Read the model definition and answer for the solid it produces. Units are mm, in the model's axes. Give positions to 0.01 mm unless a question says otherwise; leave off trailing zeros. Order: outer loops, then holes, each group sorted by start corner. A loop starts at its lowest first (then second) coordinate and runs counter-clockwise, first axis right, second up.
Item 1: Given pin 1 Ø2 at (x, z) = (31.61, 18.25) entering from +Y; pin 2 Ø18 at (x, z) = (-250, 0) entering from +Y, each flat-ended and moving along its own axis, determine where each tip first touches the part or whether it passes through.
Item 2: A cutting plane is placed at B-B (y = 6.35). State how many separate pieces and enclosed holes the cut face has, plus the area to 3 significant figures.
Item 3: A cutting plane is placed at C-C (x = -226). Write down the section's boundary in (y, z).
Item 4: Find the intervals of material crossed by line 1 along Z through (x, y) = (-169.5, 6.4); line 2 along Z through (x, y) = (-73.5, 6.9); line 3 along Z through (x, y) = (-159.5, 7.2), in increasing order.
Item 5: A cutting plane is placed at A-A (x = 5.5). Write down the section's boundary in (y, z).
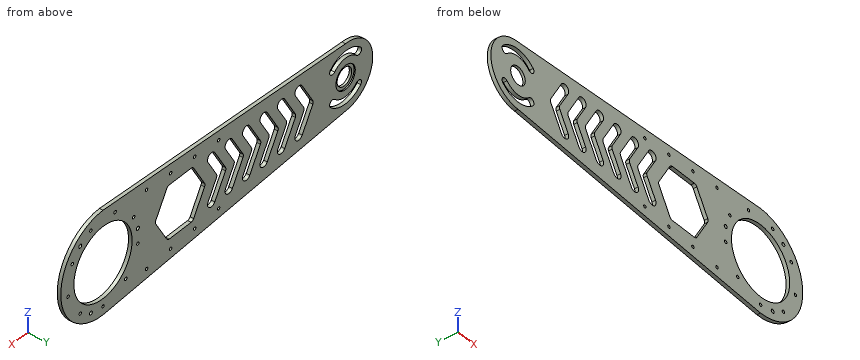
from build123d import *

# Parameters (mm, degrees)
EXTRUDE_1_DEPTH     = 3
SKETCH_3_R          = 1.25
SKETCH_3_R_2        = 30
SKETCH_3_R_3        = 1.5
CUT_EXTRUDE_1_DEPTH = 3
CUT_EXTRUDE_2_DEPTH = 3
SKETCH_5_R          = 1.25
CUT_EXTRUDE_3_DEPTH = 10
SKETCH_6_R          = 10
CUT_EXTRUDE_4_DEPTH = 1
SKETCH_7_R          = 7.5
CUT_EXTRUDE_5_DEPTH = 11


with BuildPart() as part:
    # 草图2 → 凸台-拉伸1 (new body)
    with BuildSketch(Plane(origin=(0, 5, 0), x_dir=(1, 0, 0), z_dir=(0, 1, 0))):
        with BuildLine():
            Line((-250, 28), (0, 43.5))
            ThreePointArc((0, 43.5), (43.5, 0), (0, -43.5))
            Line((0, -43.5), (-250, -28))
            ThreePointArc((-250, -28), (-278, 0), (-250, 28))
        make_face()
    extrude(amount=EXTRUDE_1_DEPTH)

    # 草图3 → 切除-拉伸1 (cut)
    with BuildSketch(Plane(origin=(0, 8, 0), x_dir=(1, 0, 0), z_dir=(0, 1, 0))):
        with Locations(Location((-250, 4, 0), (0, 0, 270))):
            Circle(SKETCH_3_R)
        with Locations(Location((-246, 0, 0), (0, 0, 270))):
            Circle(SKETCH_3_R)
        with Locations(Location((-250, -4, 0), (0, 0, 270))):
            Circle(SKETCH_3_R)
        with Locations(Location((-254, 0, 0), (0, 0, 270))):
            Circle(SKETCH_3_R)
        with Locations(Location((0, 0, 0), (0, 0, 270))):
            Circle(SKETCH_3_R_2)
        with Locations(Location((0, 36.5, 0), (0, 0, 270))):
            Circle(SKETCH_3_R)
        with Locations(Location((12.483735231, 34.298780659, 0), (0, 0, 270))):
            Circle(SKETCH_3_R_3)
        with Locations(Location((23.461747754, 27.960622174, 0), (0, 0, 270))):
            Circle(SKETCH_3_R)
        with Locations(Location((-23.461747754, 27.960622174, 0), (0, 0, 270))):
            Circle(SKETCH_3_R)
        with Locations(Location((-35.945482985, 6.338158485, 0), (0, 0, 270))):
            Circle(SKETCH_3_R)
        with Locations(Location((-35.945482985, -6.338158485, 0), (0, 0, 270))):
            Circle(SKETCH_3_R_3)
        with Locations(Location((-31.609927238, -18.25, 0), (0, 0, 270))):
            Circle(SKETCH_3_R)
        with Locations(Location((-12.483735231, -34.298780659, 0), (0, 0, 270))):
            Circle(SKETCH_3_R)
        with Locations(Location((12.483735231, -34.298780659, 0), (0, 0, 270))):
            Circle(SKETCH_3_R)
        with Locations(Location((23.461747754, -27.960622174, 0), (0, 0, 270))):
            Circle(SKETCH_3_R_3)
        with Locations(Location((31.609927238, -18.25, 0), (0, 0, 270))):
            Circle(SKETCH_3_R)
        with Locations(Location((35.945482985, 6.338158485, 0), (0, 0, 270))):
            Circle(SKETCH_3_R)
        with BuildLine():
            ThreePointArc((-265.553651429, 15.553651429), (-265.553651429, 11.316406256), (-261.316406256, 11.316406256))
            ThreePointArc((-261.316406256, 11.316406256), (-250, 16.003815204), (-238.683593744, 11.316406256))
            ThreePointArc((-238.683593744, 11.316406256), (-234.446348571, 11.316406256), (-234.446348571, 15.553651429))
            ThreePointArc((-234.446348571, 15.553651429), (-250, 21.996184796), (-265.553651429, 15.553651429))
        make_face()
        with BuildLine():
            ThreePointArc((-261.316406256, -11.316406256), (-250, -16.003815204), (-238.683593744, -11.316406256))
            ThreePointArc((-238.683593744, -11.316406256), (-234.446348571, -11.316406256), (-234.446348571, -15.553651429))
            ThreePointArc((-234.446348571, -15.553651429), (-250, -21.996184796), (-265.553651429, -15.553651429))
            ThreePointArc((-265.553651429, -15.553651429), (-265.553651429, -11.316406256), (-261.316406256, -11.316406256))
        make_face()
    extrude(amount=-CUT_EXTRUDE_1_DEPTH, mode=Mode.SUBTRACT)

    # 草图4 → 切除-拉伸2 (cut)
    with BuildSketch(Plane(origin=(0, 8, 0), x_dir=(1, 0, 0), z_dir=(0, 1, 0))):
        with BuildLine():
            Line((-216.23889617, 1.5), (-205.267472927, 20.503062488))
            ThreePointArc((-205.267472927, 20.503062488), (-199.762485666, 21.978119379), (-198.287428775, 16.473132117))
            Line((-198.287428775, 16.473132117), (-206.932170633, 1.5))
            ThreePointArc((-206.932170633, 1.5), (-207.334094422, 0), (-206.932170633, -1.5))
            Line((-206.932170633, -1.5), (-198.287428775, -16.473132117))
            ThreePointArc((-198.287428775, -16.473132117), (-199.762485666, -21.978119379), (-205.267472927, -20.503062488))
            Line((-205.267472927, -20.503062488), (-216.23889617, -1.5))
            ThreePointArc((-216.23889617, -1.5), (-216.640819958, 0), (-216.23889617, 1.5))
        make_face()
        with BuildLine():
            Line((-54.444025551, 1.5), (-65.7023558, 21))
            ThreePointArc((-65.7023558, 21), (-66.800432012, 22.098076211), (-68.300432012, 22.5))
            Line((-68.300432012, 22.5), (-90.81709251, 22.5))
            ThreePointArc((-90.81709251, 22.5), (-92.31709251, 22.098076211), (-93.415168722, 21))
            Line((-93.415168722, 21), (-104.673498971, 1.5))
            ThreePointArc((-104.673498971, 1.5), (-105.075422759, 0), (-104.673498971, -1.5))
            Line((-104.673498971, -1.5), (-93.415168722, -21))
            ThreePointArc((-93.415168722, -21), (-92.31709251, -22.098076211), (-90.81709251, -22.5))
            Line((-90.81709251, -22.5), (-68.300432012, -22.5))
            ThreePointArc((-68.300432012, -22.5), (-66.800432012, -22.098076211), (-65.7023558, -21))
            Line((-65.7023558, -21), (-54.444025551, -1.5))
            ThreePointArc((-54.444025551, -1.5), (-54.042101763, 0), (-54.444025551, 1.5))
        make_face()
        with BuildLine():
            Line((-188.932170633, -1.5), (-180.287428775, -16.473132117))
            ThreePointArc((-180.287428775, -16.473132117), (-181.762485666, -21.978119379), (-187.267472927, -20.503062488))
            Line((-187.267472927, -20.503062488), (-198.23889617, -1.5))
            ThreePointArc((-198.23889617, -1.5), (-198.640819958, 0), (-198.23889617, 1.5))
            Line((-198.23889617, 1.5), (-187.267472927, 20.503062488))
            ThreePointArc((-187.267472927, 20.503062488), (-181.762485666, 21.978119379), (-180.287428775, 16.473132117))
            Line((-180.287428775, 16.473132117), (-188.932170633, 1.5))
            ThreePointArc((-188.932170633, 1.5), (-189.334094422, 0), (-188.932170633, -1.5))
        make_face()
        with BuildLine():
            Line((-170.932170633, -1.5), (-162.287428775, -16.473132117))
            ThreePointArc((-162.287428775, -16.473132117), (-163.762485666, -21.978119379), (-169.267472927, -20.503062488))
            Line((-169.267472927, -20.503062488), (-180.23889617, -1.5))
            ThreePointArc((-180.23889617, -1.5), (-180.640819958, 0), (-180.23889617, 1.5))
            Line((-180.23889617, 1.5), (-169.267472927, 20.503062488))
            ThreePointArc((-169.267472927, 20.503062488), (-163.762485666, 21.978119379), (-162.287428775, 16.473132117))
            Line((-162.287428775, 16.473132117), (-170.932170633, 1.5))
            ThreePointArc((-170.932170633, 1.5), (-171.334094422, 0), (-170.932170633, -1.5))
        make_face()
        with BuildLine():
            Line((-152.932170633, -1.5), (-144.287428775, -16.473132117))
            ThreePointArc((-144.287428775, -16.473132117), (-145.762485666, -21.978119379), (-151.267472927, -20.503062488))
            Line((-151.267472927, -20.503062488), (-162.23889617, -1.5))
            ThreePointArc((-162.23889617, -1.5), (-162.640819958, 0), (-162.23889617, 1.5))
            Line((-162.23889617, 1.5), (-151.267472927, 20.503062488))
            ThreePointArc((-151.267472927, 20.503062488), (-145.762485666, 21.978119379), (-144.287428775, 16.473132117))
            Line((-144.287428775, 16.473132117), (-152.932170633, 1.5))
            ThreePointArc((-152.932170633, 1.5), (-153.334094422, 0), (-152.932170633, -1.5))
        make_face()
        with BuildLine():
            Line((-134.932170633, -1.5), (-126.287428775, -16.473132117))
            ThreePointArc((-126.287428775, -16.473132117), (-127.762485666, -21.978119379), (-133.267472927, -20.503062488))
            Line((-133.267472927, -20.503062488), (-144.23889617, -1.5))
            ThreePointArc((-144.23889617, -1.5), (-144.640819958, 0), (-144.23889617, 1.5))
            Line((-144.23889617, 1.5), (-133.267472927, 20.503062488))
            ThreePointArc((-133.267472927, 20.503062488), (-127.762485666, 21.978119379), (-126.287428775, 16.473132117))
            Line((-126.287428775, 16.473132117), (-134.932170633, 1.5))
            ThreePointArc((-134.932170633, 1.5), (-135.334094422, 0), (-134.932170633, -1.5))
        make_face()
        with BuildLine():
            Line((-116.932170633, -1.5), (-108.287428775, -16.473132117))
            ThreePointArc((-108.287428775, -16.473132117), (-109.762485666, -21.978119379), (-115.267472927, -20.503062488))
            Line((-115.267472927, -20.503062488), (-126.23889617, -1.5))
            ThreePointArc((-126.23889617, -1.5), (-126.640819958, 0), (-126.23889617, 1.5))
            Line((-126.23889617, 1.5), (-115.267472927, 20.503062488))
            ThreePointArc((-115.267472927, 20.503062488), (-109.762485666, 21.978119379), (-108.287428775, 16.473132117))
            Line((-108.287428775, 16.473132117), (-116.932170633, 1.5))
            ThreePointArc((-116.932170633, 1.5), (-117.334094422, 0), (-116.932170633, -1.5))
        make_face()
    extrude(amount=-CUT_EXTRUDE_2_DEPTH, mode=Mode.SUBTRACT)

    # 草图5 → 切除-拉伸3 (cut)
    with BuildSketch(Plane(origin=(0, 8, 0), x_dir=(1, 0, 0), z_dir=(0, 1, 0))):
        with Locations(Location((-44.941689831, 32.96361523, 0), (0, 0, 270))):
            Circle(SKETCH_5_R)
        with Locations(Location((-69.702891128, 31.42842075, 0), (0, 0, 270))):
            Circle(SKETCH_5_R)
        with Locations(Location((-119.225293723, 28.358031789, 0), (0, 0, 270))):
            Circle(SKETCH_5_R)
        with Locations(Location((-94.464092426, 29.89322627, 0), (0, 0, 270))):
            Circle(SKETCH_5_R)
        with Locations(Location((-44.941689831, -32.96361523, 0), (0, 0, 270))):
            Circle(SKETCH_5_R)
        with Locations(Location((-69.702891128, -31.42842075, 0), (0, 0, 270))):
            Circle(SKETCH_5_R)
        with Locations(Location((-94.464092426, -29.89322627, 0), (0, 0, 270))):
            Circle(SKETCH_5_R)
        with Locations(Location((-119.225293723, -28.358031789, 0), (0, 0, 270))):
            Circle(SKETCH_5_R)
    extrude(amount=-CUT_EXTRUDE_3_DEPTH, mode=Mode.SUBTRACT)

    # 草图6 → 切除-拉伸4 (cut)
    with BuildSketch(Plane(origin=(0, 8, 0), x_dir=(1, 0, 0), z_dir=(0, 1, 0))):
        with Locations(Location((-250, 0, 0), (0, 0, 270))):
            Circle(SKETCH_6_R)
    extrude(amount=-CUT_EXTRUDE_4_DEPTH, mode=Mode.SUBTRACT)

    # 草图7 → 切除-拉伸5 (cut)
    with BuildSketch(Plane(origin=(0, 7, 0), x_dir=(1, 0, 0), z_dir=(0, 1, 0))):
        with Locations(Location((-250, 0, 0), (0, 0, 270))):
            Circle(SKETCH_7_R)
    extrude(amount=-CUT_EXTRUDE_5_DEPTH, mode=Mode.SUBTRACT)


solid = part.part
Response values:
1. pin 1: passes through
1. pin 2: stops at y = 7
2. separate pieces: 1
2. enclosed holes: 31
2. area: 14,400 mm2
3. outline: (5, -29.49) - (8, -29.49) - (8, 29.49) - (5, 29.49) - close
4. line 1: z = -32.99 to -20.1, -3.98 to 3.98, 20.1 to 32.99
4. line 2: z = -38.94 to -22.5, 22.5 to 38.94
4. line 3: z = -33.61 to -6.24, 6.24 to 33.61
5. outline: (5, -43.15) - (8, -43.15) - (8, -29.49) - (5, -29.49) - close; (5, 29.49) - (8, 29.49) - (8, 43.15) - (5, 43.15) - close
